Could you check a few things on this model? Use its own coordinates, in mm. A direction names the side the tool comes from. Give positions to 0.01 mm unless a question says otherwise; leave off trailing zeros. Order: outer loops, then holes, each group sorted by start corner. A loop starts at its lowest first (then second) coordinate and runs counter-clockwise, first axis right, second up.
from build123d import *

# Parameters (mm, degrees)
SKETCH1_R           = 2.5
BOSS_EXTRUDE1_DEPTH = 62.5
SKETCH1_3_R         = 2
BOSS_EXTRUDE2_DEPTH = 1
SKETCH5_R           = 1
BOSS_EXTRUDE3_DEPTH = 1
SKETCH6_R           = 2
BOSS_EXTRUDE4_DEPTH = 1
SKETCH12_R          = 1.65
CUT_EXTRUDE1_DEPTH  = 5


with BuildPart() as part:
    # Sketch1 → Boss-Extrude1 (new body)
    with BuildSketch(Plane(origin=(0, 0, 0), x_dir=(1, 0, 0), z_dir=(0, 1, 0))):
        with Locations((-0.522013312, 0.511138034)):
            Circle(SKETCH1_R)
    extrude(amount=BOSS_EXTRUDE1_DEPTH)

    # Sketch1<3> → Boss-Extrude2 (add)
    with BuildSketch(Plane(origin=(0, 0, 0), x_dir=(1, 0, 0), z_dir=(0, 1, 0))):
        with Locations((-0.522013312, 0.511138034)):
            Circle(SKETCH1_3_R)
    extrude(amount=BOSS_EXTRUDE2_DEPTH)

    # Sketch5 → Boss-Extrude3 (add)
    with BuildSketch(Plane.XZ):
        with Locations((-0.522013312, -0.511138034)):
            Circle(SKETCH5_R)
    extrude(amount=BOSS_EXTRUDE3_DEPTH)

    # Sketch6 → Boss-Extrude4 (add)
    with BuildSketch(Plane.XZ.offset(1)):
        with Locations((-0.522013312, -0.511138034)):
            Circle(SKETCH6_R)
    extrude(amount=BOSS_EXTRUDE4_DEPTH)

    # Sketch12 → Cut-Extrude1 (cut)
    with BuildSketch(Plane(origin=(0, 62.5, 0), x_dir=(1, 0, 0), z_dir=(0, 1, 0))):
        with Locations((-0.522013312, 0.511138034)):
            Circle(SKETCH12_R)
    extrude(amount=-CUT_EXTRUDE1_DEPTH, mode=Mode.SUBTRACT)


solid = part.part
Item 1: Imagine slicing it at A-A on x = -0.6. List the corners of the cut face in (y, z) for me, then the cut area to 3 significant figures.
Findings:
outline: (-2, -2.51) - (-1, -2.51) - (-1, -1.51) - (0, -1.51) - (0, -3.01) - (62.5, -3.01) - (62.5, -2.16) - (57.5, -2.16) - (57.5, 1.14) - (62.5, 1.14) - (62.5, 1.99) - (0, 1.99) - (0, 0.49) - (-1, 0.49) - (-1, 1.49) - (-2, 1.49) - close
area: 302 mm2
Item 2: We'd pull the mould along Y, two halves only. Please class faces 1 (the flat face through (-1, -2, 0)), 2 (the cylindrical face through (-0.65, -0.49, 0.48)), 3 (the flat face through (-1, 57.5, -1)): +Y half, -Y half, draft (parallel to the pull), parting line (faces both ways), or undercut.
Findings:
face 1: -Y half
face 2: undercut
face 3: +Y half
Item 3: For pin 1 (1 mm diameter, centred on y = 12.5, z = -2.5, fed in from -X); pin 2 (3 mm diameter, centred on x = -0.52, z = -0.51, fed in from +Y); pin 3 (2 mm diameter, centred on x = -2, y = 6.5, fed in from -Z) (3 decimals), each with a flat end and sliding along its axis, tell me the tip position at first contact or that it passes through.
Findings:
pin 1: stops at x = -2.53
pin 2: stops at y = 57.5
pin 3: stops at z = -2.965
Item 4: For faces 4 (the cylindrical face through (1.325, -1.493, -1.277)), 5 (the flat face through (1, 0, -1)), 6 (the cylindrical face through (1.002, 60.035, 0.121)), which set-ups out of +Z, -Z, +X, -X, +Y, -Y let a thin tool reach every point of the face, with its end or its side?
Findings:
face 4: -Y
face 5: none
face 6: +Y
Item 5: Imagine slicing it at B-B on y = 43.5. List the corners of the cut face in (x, z) for me.
Findings:
outline: circle Ø5 at (-0.52, -0.51)
Item 6: Please list where these lines run through material, in increasing order: line 1 along Y through (x, z) = (-0.3, -2); line 2 along Y through (x, z) = (-2.3, 0.2); line 3 along X through (y, z) = (50.5, -0.35).
Findings:
line 1: y = -2 to -1, 0 to 57.5
line 2: y = -2 to -1, 0 to 62.5
line 3: x = -3.02 to 1.97
